from build123d import *

# Parameters (mm, degrees)
BOSS_EXTRUDE1_DEPTH = 508
BOSS_EXTRUDE2_DEPTH = 3.175
SKETCH3_W           = 438.15
SKETCH3_H           = 231.775
BOSS_EXTRUDE3_DEPTH = 3.175


with BuildPart() as part:
    # Sketch1 → Boss-Extrude1 (new body)
    with BuildSketch(Plane.XY):
        Polygon((0, 0), (3.175, 0), (3.175, 101.6), (434.975, 101.6), (434.975, -127), (438.15, -127), (438.15, 104.775), (0, 104.775), align=None)
    extrude(amount=BOSS_EXTRUDE1_DEPTH)

    # Sketch2 → Boss-Extrude2 (add)
    with BuildSketch(Plane.ZY):
        with BuildLine():
            Line((139.7, -76.2), (165.1, -76.2))
            Line((165.1, -76.2), (165.1, -127))
            Line((165.1, -127), (508, -127))
            Line((508, -127), (508, -76.2))
            Line((508, -76.2), (508, 0))
            Line((508, 0), (63.5, 0))
            ThreePointArc((63.5, 0), (117.381536726, -22.318463274), (139.7, -76.2))
        make_face()
    extrude(amount=-BOSS_EXTRUDE2_DEPTH)

    # Sketch3 → Boss-Extrude3 (add)
    with BuildSketch(Plane.XY.offset(508)):
        with Locations((219.075, -11.1125)):
            Rectangle(SKETCH3_W, SKETCH3_H)
    extrude(amount=-BOSS_EXTRUDE3_DEPTH)


solid = part.part
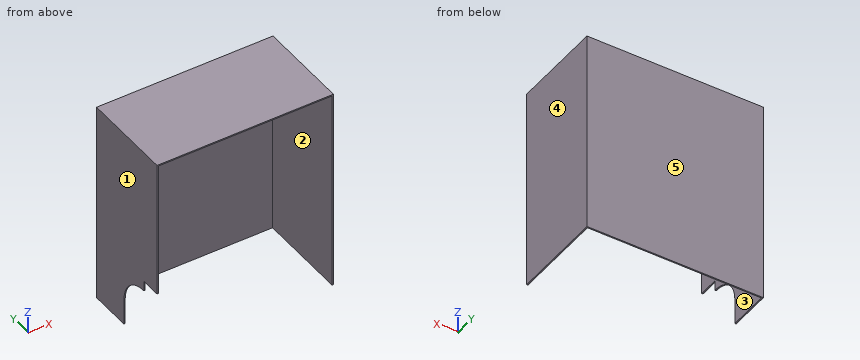
Input: part model. Units: mm. Frame: model coordinates. Face numbers are marked on the shaded views. A direction names the side the tool comes from. Round coordinates to 2 decimals unless told otherwise and drop trailing zeros. Loops run counter-clockwise (first coordinate to the right, second up) from the corner with the lowest first, then second, coordinate; pieces in that order, holes last. Notation, with made-up numbers: (-37.75, 35.25) -> (-11.75, 35.25) arc R27 cw to (-11.75, 74.25) -> close; hole circle Ø6 at (43.25, -16.75). An arc over 180 degrees is marked (long way). Answer as a JSON object with one key per item and string values. Group by question number.
1) Ray query, L1, parallel to X at y = 44.5, z = 77.5 (3 decimals); L2, parallel to Z at x = 347, y = -42 (3 decimals). Return the intervals inside material, ascending.
2) Pin query (flat end, axial travel): pin 1 (2 mm diameter, centred on x = 314, y = -86.5, fed in from -Z) (3 decimals); pin 2 (2.5 mm diameter, centred on x = 2, z = 148, fed in from -Y); pin 3 (3.5 mm diameter, centred on x = 1, z = 16, fed in from -Y). Return the tip coordinate at first contact, or that it passes through.
3) Reachability of the marked faces 1 and 2 from +Z, -Z, +X, -X, +Y, -Y: full face, straight path, thin tool, end or side. Return the list, or none.
4) Section query C-C on x = 200. Output: boundary loops of the cut face in (y, z) (3 decimals).
5) Draft query along X for the marked faces 3, 4 and 5. Return one class per face: +X half, -X half, draft (parallel to the pull), parting line (faces both ways), or undercut.
6) Section query A-A on y = 89.5. Output: boundary loops of the cut face in (x, z) (3 decimals).
7) Section query B-B on z = 316. Output: boundary loops of the cut face in (x, y) (3 decimals), plus the area to 3 significant figures.
Reply:
{
 "1": {"L1": "x = 0 to 3.175, 434.975 to 438.15", "L2": "z = 504.825 to 508"},
 "2": {"pin 1": "stops at z = 504.825", "pin 2": "stops at y = -76.2", "pin 3": "stops at y = 0"},
 "3": {"face 1": "+Z, -Z, -X, +Y, -Y", "face 2": "-Z, -Y"},
 "4": {"outline": "(-127, 504.825) -> (101.6, 504.825) -> (101.6, 0) -> (104.775, 0) -> (104.775, 508) -> (-127, 508) -> close"},
 "5": {"face 3": "undercut", "face 4": "+X half", "face 5": "draft"},
 "6": {"outline": "(0, 0) -> (3.175, 0) -> (3.175, 504.825) -> (434.975, 504.825) -> (434.975, 0) -> (438.15, 0) -> (438.15, 508) -> (0, 508) -> close"},
 "7": {"outline": "(0, -127) -> (3.175, -127) -> (3.175, 101.6) -> (434.975, 101.6) -> (434.975, -127) -> (438.15, -127) -> (438.15, 104.775) -> (0, 104.775) -> close", "area": "2,840 mm2"}
}
